The drawing under review shows one solid part. Ordinate dimensions are in mm from its lowest x, y, z. A direction names the side the tool comes from. Coordinates: 2 decimals unless noted, no trailing zeros. Order: outer loops, then holes, each group sorted by start corner. A loop starts at its lowest first (then second) coordinate and runs counter-clockwise, first axis right, second up. Notation, with made-up numbers: M -4,46 L 28,46 A25 ccw 28,60 Z; hole C 69.5,9 d10. An arc over 180 degrees is marked long. Answer as a JSON object with one key per item and string values.
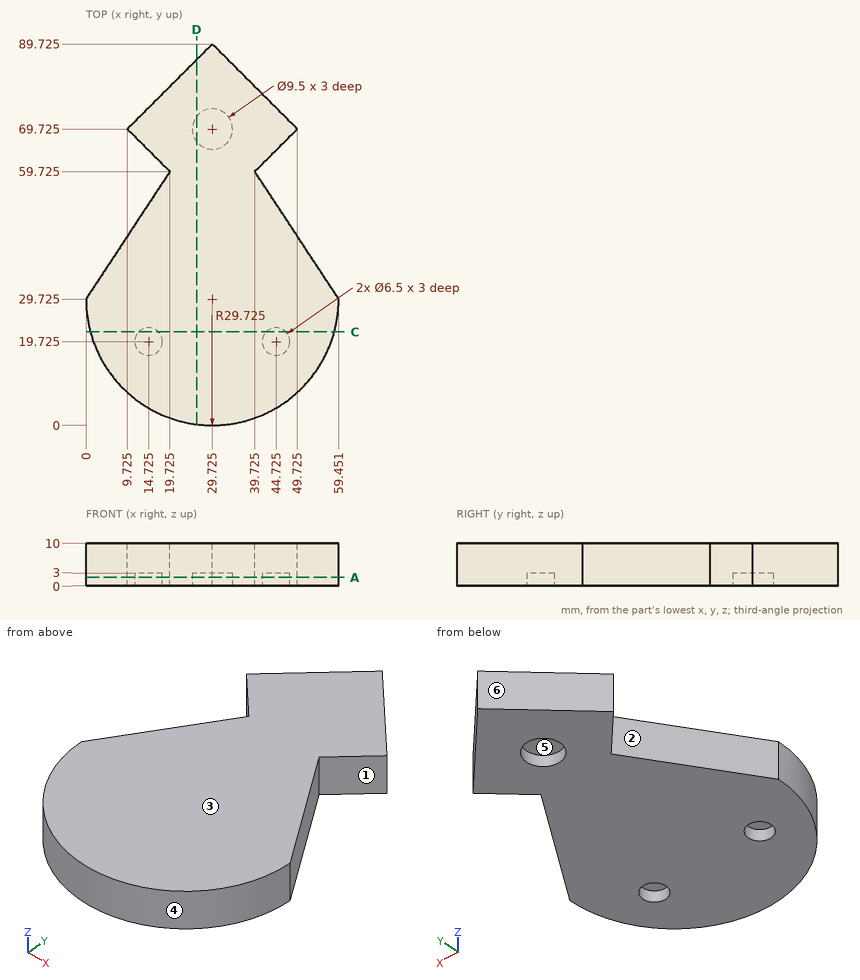
1) Mouldability with a two-part tool opening along Y and no side actions: class the marked faces 1, 2, 3 and 4 as released by +Y, released by -Y, zero draft, split by the parting line, or undercut.
Taken from the geometry:
{"face 1": "undercut", "face 2": "undercut", "face 3": "zero draft", "face 4": "released by -Y"}
2) Add section C-C (y = 22). State the section outline as (x, z) points (1 decimal), and give its area (3 significant figures).
Taken from the geometry:
{"outline": "M 1,0 L 12.4,0 L 12.4,3 L 17,3 L 17,0 L 42.4,0 L 42.4,3 L 47,3 L 47,0 L 58.4,0 L 58.4,10 L 1,10 Z", "area": "546 mm2"}
3) To check wall thickness, follow L1, parallel to X at y = 22, z = 1.5 (1 decimal); L2, parallel to Z at x = 15.5, y = 18; L3, parallel to X at y = 4, z = 8.75 (1 decimal). State the ranges of each line that lie inside material, in increasing order.
Taken from the geometry:
{"L1": "x = 1 to 12.4, 17 to 42.4, 47 to 58.4", "L2": "z = 3 to 10", "L3": "x = 14.8 to 44.6"}
4) Tool access review of the marked faces 5 and 6: name each direction out of +Z, -Z, +X, -X, +Y, -Y from which nothing blocks a thin tool from reaching the whole face with its end or side.
Taken from the geometry:
{"face 5": "-Z", "face 6": "+Z, -Z, -X, +Y"}
5) Add section A-A (z = 2). Count the separate pieces of the cut face and the enclosed holes in it, and give its area (3 significant figures).
Taken from the geometry:
{"separate pieces": "1", "enclosed holes": "3", "area": "3,140 mm2"}
6) Add section D-D (x = 26). State the section outline as (y, z) points (1 decimal).
Taken from the geometry:
{"outline": "M 0.2,0 L 66.8,0 L 66.8,3 L 72.7,3 L 72.7,0 L 86,0 L 86,10 L 0.2,10 Z"}
7) Insertion check: pin 1 Ø2 at (y, z) = (65, 8.5) entering from -X; pin 2 Ø3 at (x, z) = (31.5, 1) entering from -Y; pin 3 Ø5 at (x, y) = (14.73, 19.73) entering from -Z; pin 4 Ø2 at (x, y) = (45, 78) entering from +Z. Each pin has a flat end and moves straight along its axis. Give the tip position at first contact, or say it passes through.
Taken from the geometry:
{"pin 1": "stops at x = 13.45", "pin 2": "stops at y = 0", "pin 3": "stops at z = 3", "pin 4": "passes through"}
